For this review, take the finished solid that the model builds, in its own axes (mm). A direction names the side the tool comes from. Coordinates: 2 decimals unless noted, no trailing zeros. Write each loop counter-clockwise with the first axis right and the second up, starting at its lowest first coordinate (ties: lowest second). Pieces come first, ordered by that corner, then holes. Notation, with made-up numbers: M 83,-40 L 93,-40 A28 cw 93,-6 Z; hole C 66,61.25 d10. An arc over 180 degrees is marked long. Return JSON: item names as keys, results as strings.
```python
from build123d import *

# Parameters (mm, degrees)
PAD001_DEPTH         = 19
SKETCH004_R          = 14
POCKET_DEPTH         = 0.001
POCKET_DEPTH_BACK    = 19.001
POCKET001_DEPTH      = 14
FILLET_R             = 5
SKETCH012_W          = 12
SKETCH012_H          = 12
POCKET003_DEPTH      = 1.5
SKETCH013_W          = 1
SKETCH013_H          = 2
POCKET004_DEPTH      = 19.001
POCKET004_DEPTH_BACK = 0.001
SKETCH016_W          = 10
SKETCH016_H          = 3
POCKET007_DEPTH      = 75.001


with BuildPart() as part:
    # Sketch005 → Pad001 (new body)
    with BuildSketch(Plane.XY):
        with BuildLine():
            Line((119, 31.35), (119, 117.813456))
            ThreePointArc((119, 117.813456), (115.825, 123.312717), (109.475, 123.312717))
            Line((109.475, 123.312717), (91.368603, 112.858984))
            ThreePointArc((82.694341, 115.183245), (86.550102, 112.224616), (91.368603, 112.858984))
            Line((82.694341, 115.183245), (69.044341, 138.825739))
            ThreePointArc((71.368603, 147.5), (68.409974, 143.64424), (69.044341, 138.825739))
            Line((71.368603, 147.5), (119, 175))
            Line((119, 175), (173.65, 175))
            ThreePointArc((180, 168.65), (178.140128, 173.140128), (173.65, 175))
            Line((180, 168.65), (180, 31.35))
            ThreePointArc((173.65, 25), (178.140128, 26.859872), (180, 31.35))
            Line((173.65, 25), (125.35, 25))
            ThreePointArc((119, 31.35), (120.859872, 26.859872), (125.35, 25))
        make_face()
    extrude(amount=PAD001_DEPTH)

    # Sketch004 → Pocket (cut, two sides)
    with BuildSketch(Plane.XY) as pocket_sk:
        with Locations((152, 124.5)):
            Circle(SKETCH004_R)
        with Locations((152, 66.5)):
            Circle(SKETCH004_R)
    extrude(amount=-POCKET_DEPTH, mode=Mode.SUBTRACT)
    extrude(pocket_sk.sketch, amount=POCKET_DEPTH_BACK, mode=Mode.SUBTRACT)

    # Sketch006 → Pocket001 (cut)
    with BuildSketch(Plane.XY):
        with BuildLine():
            Line((73.868603, 143.169873), (120.339746, 170))
            Line((120.339746, 170), (165, 170))
            ThreePointArc((165, 170), (167.928932, 162.928932), (175, 160))
            Line((175, 160), (175, 30))
            Line((175, 30), (134, 30))
            ThreePointArc((134, 30), (131.071068, 37.071068), (124, 40))
            Line((124, 40), (124, 137.472233))
            Line((124, 137.472233), (88.868603, 117.189111))
            Line((88.868603, 117.189111), (73.868603, 143.169873))
        make_face()
    extrude(amount=POCKET001_DEPTH, mode=Mode.SUBTRACT)

    # Fillet
    fillet_edges = [part.edges().sort_by_distance(p)[0] for p in [
        (119, 74.581728, 19),
    ]]
    fillet(fillet_edges, radius=FILLET_R)

    # Sketch012 → Pocket003 (cut, symmetric)
    with BuildSketch(Plane.XY.offset(19)):
        with Locations((125, 161)):
            Rectangle(SKETCH012_W, SKETCH012_H)
    extrude(amount=POCKET003_DEPTH, both=True, mode=Mode.SUBTRACT)

    # Sketch013 → Pocket004 (cut, two sides)
    with BuildSketch(Plane.XY.offset(19)) as pocket004_sk:
        with Locations((119.5, 163.333333)):
            Rectangle(SKETCH013_W, SKETCH013_H)
        with Locations((130.5, 163.333333)):
            Rectangle(SKETCH013_W, SKETCH013_H)
        with Locations((119.5, 158.666667)):
            Rectangle(SKETCH013_W, SKETCH013_H)
        with Locations((130.5, 158.666667)):
            Rectangle(SKETCH013_W, SKETCH013_H)
    extrude(amount=-POCKET004_DEPTH, mode=Mode.SUBTRACT)
    extrude(pocket004_sk.sketch, amount=POCKET004_DEPTH_BACK, mode=Mode.SUBTRACT)

    # Sketch016 → Pocket007 (cut, through all)
    with BuildSketch(Plane.XZ.offset(-100)):
        with Locations((152, 1.5)):
            Rectangle(SKETCH016_W, SKETCH016_H)
    extrude(amount=-POCKET007_DEPTH, mode=Mode.SUBTRACT)


solid = part.part
```
1. Wall thickness on L1, parallel to X at y = 47.5, z = 6.5; L2, parallel to Y at x = 140, z = 8.75; L3, parallel to Y at x = 152, z = 16.05: over which ranges is each line inside the solid? List them lowest first. Write a range as from..to.
Checks:
{"L1": "119..124, 175..180", "L2": "25..30, 170..175", "L3": "25.44..52.5, 80.5..110.5, 138.5..174.56"}
2. Clearance check with flat-ended pins moving along their axes: pin 1 Ø8 at (x, y) = (155.5, 159) entering from -Z; pin 2 Ø11 at (y, z) = (65.5, 8) entering from -X; pin 3 Ø1.2 at (x, z) = (123, 18.5) entering from -Y. State where each tip first meets the part, or that it passes through.
Checks:
{"pin 1": "z = 14", "pin 2": "x = 119", "pin 3": "y = 27.47"}
3. We need section B-B (x = 152). State the section outline as (y, z) points.
Checks:
{"outline": "M 25,0 L 30,0 L 30,14 L 52.5,14 L 52.5,19 L 30,19 A5 ccw 25,14 Z; M 80.5,14 L 110.5,14 L 110.5,19 L 80.5,19 Z; M 138.5,14 L 170,14 L 170,3 L 175,3 L 175,14 A5 ccw 170,19 L 138.5,19 Z"}
4. Draft analysis for pull direction Y (two halves, no side actions). For faces 4 (the face through (75.965, 126.839, 6.902)), 5 (the face through (147, 172, 1)), 6 (the face through (136, 117, 14)), state which applies: +Y half, -Y half, draft (parallel to the pull), parting line (faces both ways), or undercut.
Checks:
{"face 4": "-Y half", "face 5": "draft", "face 6": "undercut"}
5. We need section D-D (y = 50.5). State the section outline as (x, z) points.
Checks:
{"outline": "M 119,0 L 124,0 L 124,14 L 175,14 L 175,0 L 180,0 L 180,14 A5 ccw 175,19 L 124,19 A5 ccw 119,14 Z"}
6. We need section A-A (y = 66.5). State the section outline as (x, z) points, plus the area to 3 significant figures.
Checks:
{"outline": "M 119,0 L 124,0 L 124,14 L 138,14 L 138,19 L 124,19 A5 ccw 119,14 Z; M 166,14 L 175,14 L 175,0 L 180,0 L 180,14 A5 ccw 175,19 L 166,19 Z", "area": "294 mm2"}
7. For faces 1 (the face through (119, 161, 18)), 2 (the face through (106.68, 127.473, 6.902)), 3 (the face through (100.55, 118.16, 6.9)), list the 3-axis set-ups (+Z, -Z, +X, -X, +Y, -Y) from which the entire face can be reached by the end or side of a thin tool; tool diameter is ignored.
Checks:
{"face 1": "+Z", "face 2": "-Z", "face 3": "+Z, -Z, -Y"}
8. We need section C-C (z = 7). State the section outline as (x, y) points (3 decimals).
Checks:
{"outline": "M 69.044,138.826 L 82.694,115.183 A6.35 ccw 91.369,112.859 L 109.475,123.313 A6.35 cw 119,117.813 L 119,31.35 A6.35 ccw 125.35,25 L 173.65,25 A6.35 ccw 180,31.35 L 180,168.65 A6.35 ccw 173.65,175 L 119,175 L 71.369,147.5 A6.35 ccw Z; hole M 73.869,143.17 L 88.869,117.189 L 124,137.472 L 124,40 A10 cw 134,30 L 175,30 L 175,160 A10 cw 165,170 L 120.34,170 Z"}
